Verification items for the finished model (mm, model axes). Face numbers are marked on the shaded views. A direction names the side the tool comes from. Give positions to 0.01 mm unless a question says otherwise; leave off trailing zeros. Write each loop counter-clockwise with the first axis right and the second up, starting at its lowest first coordinate (ties: lowest second). Pieces come first, ordered by that corner, then holes. Notation, with made-up numbers: (-9.75, 47) - (31.25, 47) arc R14 ccw to (31.25, 54) - close; hole circle Ø11 at (41, 26). An arc over 180 degrees is marked (long way). Answer as a JSON object with one key per item and string values. Group by question number.
Item 1: Go/stop test with flat-tipped pins: pin 1 (1.5 mm diameter, centred on x = 11.5, z = 6.5, fed in from -Y); pin 2 (4.5 mm diameter, centred on y = -4.5, z = 6, fed in from -X); pin 3 (4.5 mm diameter, centred on y = 10, z = 6.5, fed in from +X). Record where each tip stops, or that it passes through.
Item 2: Sectioned sample at C-C, the plane z = 7. Record the boundary of the cut face in (x, y).
Item 3: Tool access check on the marked faces 3 and 4. Record the directions out of +Z, -Z, +X, -X, +Y, -Y that give a thin tool (end or side, any length) a straight path to the whole face; none if there is none.
Item 4: Scan lines: line 1 along X through (y, z) = (-1, 4.75); line 2 along Z through (x, y) = (16, 21). Record each from-to range of solid material in increasing order. Write a range as [from, to].
Item 5: Draft check along X on the marked faces 1 and 2. Enter one of: +X half, -X half, draft (parallel to the pull), parting line (faces both ways), or undercut.
Item 6: Sectioned sample at A-A, the plane x = -16.5. Record the boundary of the cut face in (y, z).
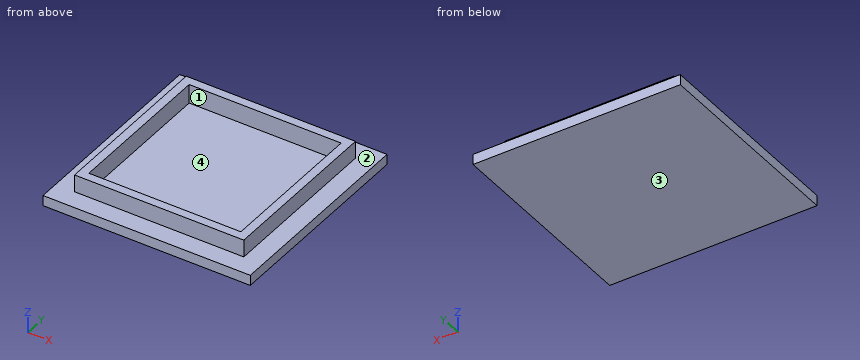
```python
from build123d import *

# Parameters (mm, degrees)
F0_W        = 60
F0_H        = 60
F1_DEPTH    = 3
F2_W        = 49
F2_H        = 49
F3_DEPTH    = 5
F4_T        = 2.5
F4_T3_DEPTH = 54
F4_T5_DEPTH = 54


# Not quite as in the source:
# - a shell that OpenCascade refuses in one call is made with other operations: the cavity is built on its own and cut out


with BuildPart() as f1:
    # F0 (on Top) → F1 (new body)
    with BuildSketch(Plane.XY):
        Rectangle(F0_W, F0_H)
    extrude(amount=F1_DEPTH)

    # F2 (on face) → F3 (join)
    with BuildSketch(Plane.XY.offset(3)):
        Rectangle(F2_W, F2_H)
    extrude(amount=F3_DEPTH)

    # F4: shell of thickness 2.5, made by hand


with BuildPart() as f4_core1:
    # F4_t2: copy of F1
    add(f1.part)

    # the walls: a layer under each face that stays
    f4_faces = [f4_core1.faces().sort_by_distance(p)[0] for p in [
        (0, -30, 1.5),
        (-30, 0, 1.5),
        (30, 0, 1.5),
        (0, 0, 0),
        (-25.7142857143, -25.7142857143, 3),
        (0, 30, 1.5),
        (0, -24.5, 5.5),
        (24.5, 0, 5.5),
        (0, 24.5, 5.5),
        (-24.5, 0, 5.5),
    ]]
    thicken(f4_faces, amount=-F4_T, mode=Mode.SUBTRACT)

    # F4_s4 → F4_t3 (cut)
    with BuildSketch(Plane.YZ.offset(-27)):
        Polygon((-24.525, 3.025), (-24.5, 0.5), (-22, 0.5), (-22, 3), align=None)
        Polygon((24.525, 3.025), (24.5, 0.5), (22, 0.5), (22, 3), align=None)
    extrude(amount=F4_T3_DEPTH, mode=Mode.SUBTRACT)

    # F4_s6 → F4_t5 (cut)
    with BuildSketch(Plane.XZ.offset(-27)):
        Polygon((24.525, 3.025), (24.5, 0.5), (22, 0.5), (22, 3), align=None)
        Polygon((-24.525, 3.025), (-24.5, 0.5), (-22, 0.5), (-22, 3), align=None)
    extrude(amount=F4_T5_DEPTH, mode=Mode.SUBTRACT)


with BuildPart() as f1_1:
    add(f1.part)

    # what is left inside the walls is the cavity
    f4_cavity = [f4_core1.part.solids().sort_by_distance(p)[0] for p in [
        (0, -7.333333, 2.525),
    ]]
    add(f4_cavity, mode=Mode.SUBTRACT)


solid = f1_1.part
```
Geometry check:
{
 "1": {"pin 1": "y = -24.5", "pin 2": "x = -24.5", "pin 3": "x = 24.5"},
 "2": {"outline": "(-24.5, -24.5) - (24.5, -24.5) - (24.5, 24.5) - (-24.5, 24.5) - close; hole (-22, -22) - (22, -22) - (22, 22) - (-22, 22) - close"},
 "3": {"face 3": "-Z, +X, -X, +Y, -Y", "face 4": "+Z"},
 "4": {"line 1": "[-24.5, -22], [22, 24.5]", "line 2": "[0, 2.5]"},
 "5": {"face 1": "undercut", "face 2": "draft"},
 "6": {"outline": "(-30, 0) - (30, 0) - (30, 3) - (24.5, 3) - (24.5, 8) - (22, 8) - (22, 2.5) - (-22, 2.5) - (-22, 8) - (-24.5, 8) - (-24.5, 3) - (-30, 3) - close"}
}
